Verification items for the finished model (mm, model axes). Round coordinates to 2 decimals unless told otherwise and drop trailing zeros. Order: outer loops, then holes, each group sorted by start corner. A loop starts at its lowest first (then second) coordinate and runs counter-clockwise, first axis right, second up.
```python
from build123d import *

# Parameters (mm, degrees)
SKETCH1_W             = 148
SKETCH1_H             = 60
SKETCH1_R             = 3.25
SKETCH1_R_2           = 5
BOSS_EXTRUDE1_DEPTH   = 6
M5X0_8_TAPPED_HOLE1_D = 4.2
M4X0_7_TAPPED_HOLE1_D = 3.3
M3X0_5_TAPPED_HOLE1_D = 2.5
CHAMFER1_SIZE         = 10
CHAMFER2_SIZE         = 3


with BuildPart() as part:
    # Sketch1 → Boss-Extrude1 (new body)
    with BuildSketch(Plane.XY):
        with Locations((20.481223922, -2.599443672)):
            Rectangle(SKETCH1_W, SKETCH1_H)
        with Locations((-34.993045897, 12.400556328)):
            Circle(SKETCH1_R, mode=Mode.SUBTRACT)
        with Locations((-4.993045897, 12.400556328)):
            Circle(SKETCH1_R, mode=Mode.SUBTRACT)
        with Locations((-34.993045897, -17.599443672)):
            Circle(SKETCH1_R, mode=Mode.SUBTRACT)
        with Locations((-4.993045897, -17.599443672)):
            Circle(SKETCH1_R, mode=Mode.SUBTRACT)
        with Locations((74.481223922, -8.599443672)):
            Circle(SKETCH1_R_2, mode=Mode.SUBTRACT)
    extrude(amount=BOSS_EXTRUDE1_DEPTH)

    # M5x0.8 Tapped Hole1 (through all)
    with Locations(Plane.XY.offset(6)):
        with Locations((74.481223922, 7.400556328), (74.481223922, -24.599443672)):
            Hole(M5X0_8_TAPPED_HOLE1_D / 2)

    # M4x0.7 Tapped Hole1 (through all)
    with Locations(Plane.XY.offset(6)):
        with Locations((89.481223922, 22.400556328), (51.481223922, -13.099443672)):
            Hole(M4X0_7_TAPPED_HOLE1_D / 2)

    # M3x0.5 Tapped Hole1 (through all)
    with Locations(Plane.XY.offset(6)):
        with Locations((0.781223922, -15.449443672), (8.781223922, -15.449443672)):
            Hole(M3X0_5_TAPPED_HOLE1_D / 2)

    # Chamfer1
    chamfer1_edges = [part.edges().sort_by_distance(p)[0] for p in [
        (94.481223922, -32.599443672, 3),
    ]]
    chamfer(chamfer1_edges, length=CHAMFER1_SIZE)

    # Chamfer2
    chamfer2_edges = [part.edges().sort_by_distance(p)[0] for p in [
        (-53.518776078, 27.400556328, 3),
        (94.481223922, 27.400556328, 3),
        (-53.518776078, -32.599443672, 3),
    ]]
    chamfer(chamfer2_edges, length=CHAMFER2_SIZE)


solid = part.part
```
1) Sectioned sample at A-A on y = -6. Record the cut outline in (x, z), then the cut area to 3 significant figures.
2) Scan lines: probe 1 along X at (y, z) = (-12, 3.45); probe 2 along X at (y, z) = (-16.5, 4.6); probe 3 along X at (y, z) = (-24, 2.1). Record each from-to range of solid material in increasing order.
3) Sectioned sample at B-B on z = 2.6. Count the separate pieces of the cut face and the enclosed holes in it, then the cut area to 3 significant figures.
Returned:
1. outline: (-53.52, 0) - (70.21, 0) - (70.21, 6) - (-53.52, 6) - close; (78.75, 0) - (94.48, 0) - (94.48, 6) - (78.75, 6) - close
1. area: 837 mm2
2. probe 1: x = -53.52 to 50.25, 52.71 to 70.82, 78.15 to 94.48
2. probe 2: x = -53.52 to -38.05, -31.93 to -8.05, -1.93 to 0.1, 1.46 to 8.1, 9.46 to 94.48
2. probe 3: x = -53.52 to 72.47, 76.49 to 93.08
3. separate pieces: 1
3. enclosed holes: 11
3. area: 8,550 mm2
